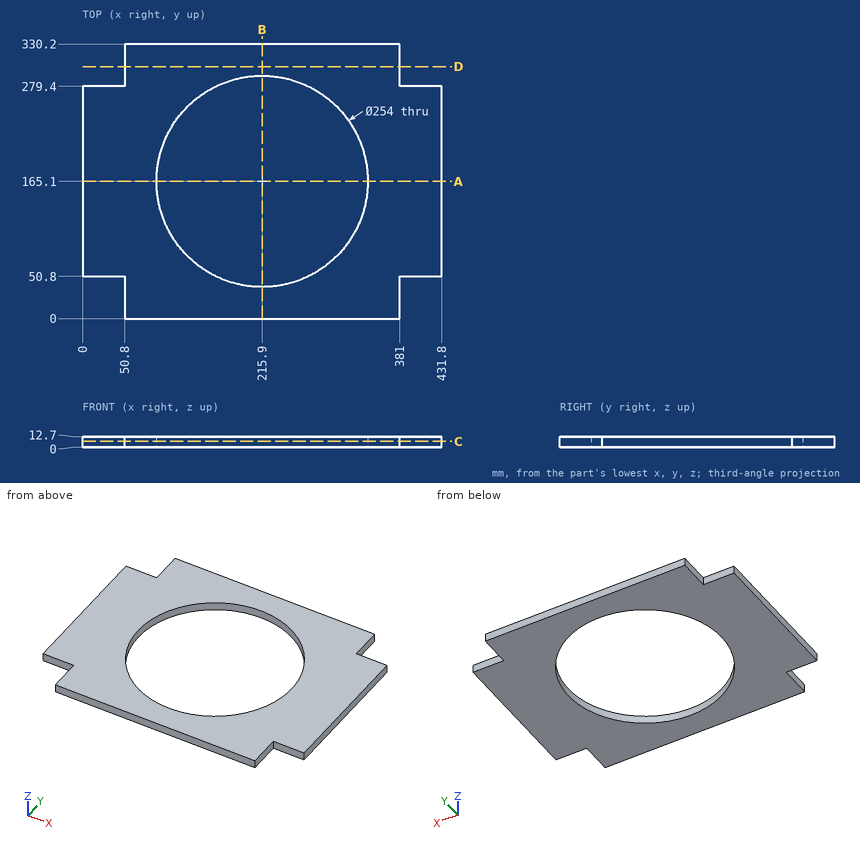
Study the drawing (mm; zero at the part's minimum x, y, z) and answer. Give positions to 0.01 mm unless a question says otherwise; leave off trailing zeros. Order: outer loops, then holes, each group sorted by start corner. A loop starts at its lowest first (then second) coordinate and runs counter-clockwise, first axis right, second up. Notation, with made-up numbers: (81, 27.5) - (139, 27.5) arc R20 cw to (139, 39.5) - close; hole circle Ø11 at (17.25, 8.25). An arc over 180 degrees is marked (long way). Answer in a Markdown table with one row per item. Add a question column.
Q1. The part is cut by section D-D (y = 303). Determine the outline of the cut face in (x, z).
Q2. Find the intervals of material crossed by line 1 along Y through (x, z) = (218, 9.25); line 2 along X through (y, z) = (314, 2.5); line 3 along Y through (x, z) = (20, 10.5), in increasing order. Write a range as [from, to].
Q3. The part is cut by section C-C (z = 7.25). Determine the outline of the cut face in (x, y).
Q4. Given P1, Ø6.5, axis at y = 314, z = 9, coming from the -X side; P2, Ø6.5, axis at y = 307.5, z = 8, coming from the +X side; P3, Ø4, axis at x = 415.5, z = 6.5, coming from the -Y side, each flat-ended and moving along its own axis, determine where each tip first touches the part or whether it passes through.
Q5. The part is cut by section B-B (x = 215.9). Determine the outline of the cut face in (y, z), then the cut area to 3 significant figures.
Q6. The part is cut by section A-A (y = 165.1). Determine the outline of the cut face in (x, z).
Determined:
| question | item | result |
|---|---|---|
| 1 | outline | (50.8, 0) - (381, 0) - (381, 12.7) - (50.8, 12.7) - close |
| 2 | line 1 | y = [0, 38.12], [292.08, 330.2] |
| 2 | line 2 | x = [50.8, 381] |
| 2 | line 3 | y = [50.8, 279.4] |
| 3 | outline | (0, 50.8) - (50.8, 50.8) - (50.8, 0) - (381, 0) - (381, 50.8) - (431.8, 50.8) - (431.8, 279.4) - (381, 279.4) - (381, 330.2) - (50.8, 330.2) - (50.8, 279.4) - (0, 279.4) - close; hole circle Ø254 at (215.9, 165.1) |
| 4 | P1 | stops at x = 50.8 |
| 4 | P2 | stops at x = 381 |
| 4 | P3 | stops at y = 50.8 |
| 5 | outline | (0, 0) - (38.1, 0) - (38.1, 12.7) - (0, 12.7) - close; (292.1, 0) - (330.2, 0) - (330.2, 12.7) - (292.1, 12.7) - close |
| 5 | area | 968 mm² |
| 6 | outline | (0, 0) - (88.9, 0) - (88.9, 12.7) - (0, 12.7) - close; (342.9, 0) - (431.8, 0) - (431.8, 12.7) - (342.9, 12.7) - close |
